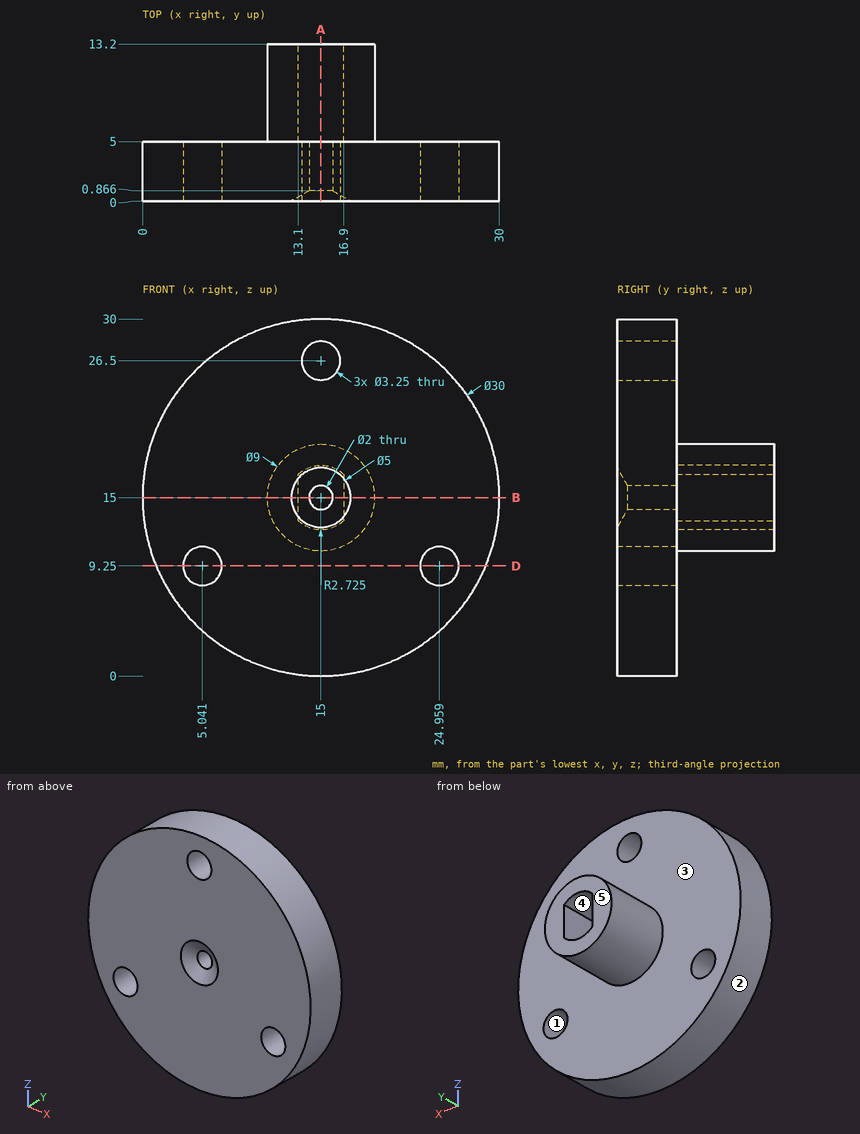
The figure shows three views and two pictorial views of one solid part (mm, origin at its lowest corner). Answer the questions. A direction names the side the tool comes from. Coordinates: 2 decimals unless noted, no trailing zeros. Order: outer loops, then holes, each group sorted by start corner. A loop starts at its lowest first (then second) coordinate and runs counter-clockwise, first axis right, second up. Notation, with made-up numbers: (-4, -19) - (20, -19) arc R19 ccw to (20, 6) - close; hole circle Ø7 at (40, 70). An arc over 180 degrees is marked (long way). Answer as a JSON object with one key per item and string values.
1. Find section B-B on z = 15. Determine the outline of the cut face in (x, y), plus the area to 3 significant figures.
Output values:
{"outline": "(0, 0) - (12.5, 0) - (14, 0.87) - (14, 5) - (13.1, 5) - (13.1, 13.2) - (10.5, 13.2) - (10.5, 5) - (0, 5) - close; (16, 0.87) - (17.5, 0) - (30, 0) - (30, 5) - (19.5, 5) - (19.5, 13.2) - (16.9, 13.2) - (16.9, 5) - (16, 5) - close", "area": "181 mm²"}
2. Consider line 1 (Z direction, x = 14.5, y = 2) (1 decimal); line 2 (Y direction, x = 21, z = 22.75); line 3 (X direction, y = 2.8, z = 26.5) (1 decimal). Determine where each line is inside the solid, lowest interval first.
Output values:
{"line 1": "z = 0 to 14.1, 15.9 to 25, 28 to 30", "line 2": "y = 0 to 5", "line 3": "x = 5.4 to 13.4, 16.6 to 24.6"}
3. Find section A-A on x = 15. Determine the outline of the cut face in (y, z) (1 decimal).
Output values:
{"outline": "(0, 0) - (5, 0) - (5, 10.5) - (13.2, 10.5) - (13.2, 12.3) - (5, 12.3) - (5, 14) - (0.9, 14) - (0, 12.5) - close; (0, 17.5) - (0.9, 16) - (5, 16) - (5, 17.7) - (13.2, 17.7) - (13.2, 19.5) - (5, 19.5) - (5, 24.9) - (0, 24.9) - close; (0, 28.1) - (5, 28.1) - (5, 30) - (0, 30) - close"}
4. A tool of negligible diameter and unlimited length cuts with its end or side. For the marked faces 4 and 5, from which of +Z, -Z, +X, -X, +Y, -Y can it reach the whole face along a straight path? Write none if from no direction.
Output values:
{"face 4": "+Y", "face 5": "+Z, -Z, +X, -X, +Y"}
5. Each of these flat-tipped pins is pushed along its axis until it touches: P1, Ø4, axis at x = 19, z = 20.5, coming from the +Y side; P2, Ø1.2, axis at y = 10, z = 14.5, coming from the -X side; P3, Ø3, axis at x = 8, y = 1.5, coming from the +Z side (1 decimal); P4, Ø4, axis at x = 6, y = 8.5, coming from the +Z side. Where does it stop, or does it pass through?
Output values:
{"P1": "stops at y = 5", "P2": "stops at x = 10.5", "P3": "stops at z = 29", "P4": "passes through"}
6. Find section D-D on z = 9.25. Determine the outline of the cut face in (x, y).
Output values:
{"outline": "(1.15, 0) - (3.42, 0) - (3.42, 5) - (1.15, 5) - close; (6.67, 0) - (23.33, 0) - (23.33, 5) - (6.67, 5) - close; (26.58, 0) - (28.85, 0) - (28.85, 5) - (26.58, 5) - close"}
7. The mould has two halves that part along X. Classify the marked faces 1, 2 and 3: +X half, -X half, draft (parallel to the pull), parting line (faces both ways), or undercut.
Output values:
{"face 1": "undercut", "face 2": "parting line", "face 3": "draft"}
